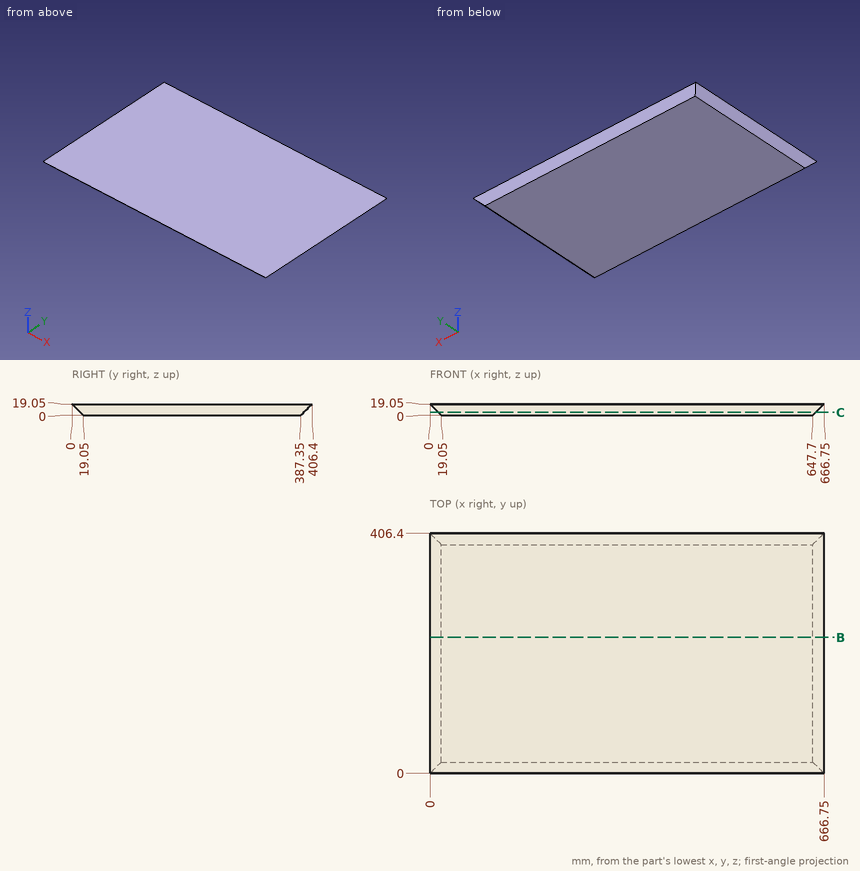
Geometry check sheet. Reference: drawing and pictorial views, mm from the part's lowest x, y, z. Give positions to 0.01 mm unless a question says otherwise; leave off trailing zeros. Write each loop counter-clockwise with the first axis right and the second up, starting at its lowest first coordinate (ties: lowest second). Pieces come first, ordered by that corner, then holes.
Item 1: Scan lines: L1, parallel to X at y = 331.5, z = 4; L2, parallel to X at y = 348.5, z = 9.75; L3, parallel to Y at x = 635, z = 3.75. Record each from-to range of solid material in increasing order.
Item 2: Cross-section at B-B (y = 230). Enter the section's corners in (x, z), and give its area (3 significant figures).
Item 3: Gauge pin test, flat ends, axial feed: pin 1 (1 mm diameter, centred on x = 75, z = 2.5, fed in from -Y); pin 2 (6 mm diameter, centred on y = 284.5, z = 15.5, fed in from +X); pin 3 (3 mm diameter, centred on y = 362.5, z = 9, fed in from -X). Record the tip position at first contact, or that the pin passes through.
Item 4: Cross-section at C-C (z = 4.75). Enter the section's corners in (x, y).
Report:
1. L1: x = 15.05 to 651.7
1. L2: x = 9.3 to 657.45
1. L3: y = 15.3 to 391.1
2. outline: (0, 19.05) - (19.05, 0) - (647.7, 0) - (666.75, 19.05) - close
2. area: 12,300 mm2
3. pin 1: stops at y = 16.05
3. pin 2: stops at x = 666.2
3. pin 3: stops at x = 8.55
4. outline: (14.3, 14.3) - (652.45, 14.3) - (652.45, 392.1) - (14.3, 392.1) - close
